Source: three-view drawing plus pictorial views. Frame: mm from the lowest corner of the part. A direction names the side the tool comes from. Give positions to 0.01 mm unless a question says otherwise; leave off trailing zeros. Loops run counter-clockwise (first coordinate to the right, second up) from the corner with the lowest first, then second, coordinate; pieces in that order, holes last. Notation, with made-up numbers: (74, 63) - (123, 63) arc R10 cw to (123, 68) - close; hole circle Ø7 at (-37, 78). An arc over 180 degrees is marked (long way). Answer as a JSON object with one key per item and string values. Group by question number.
(1) Section query B-B (y = 27.5). Return loops of the section in (x, z).
(2) Section query C-C (z = 7). Return loops of the section in (x, y).
(3) Section query D-D (x = 30). Return loops of the section in (y, z).
(4) Access query for the marked faces 1, 2, 3 and 4. Directions: +Z, -Z, +X, -X, +Y, -Y. A direction counts if a zero-diameter tool reaches every point of the face in a straight line with its end or side. Return the directions, or none.
(5) Pin query (flat end, axial travel): P1, Ø3, axis at y = 4, z = 5.5, coming from the +X side; P2, Ø1.5, axis at x = 26.5, z = 10.5, coming from the +Y side; P3, Ø6, axis at x = 30, y = 7.5, coming from the -Z side; P4, Ø3, axis at x = 16, z = 5, coming from the -Y side. Return the tip coordinate at first contact, or that it passes through.
(6) Mould query, pull axis X, two halves, no side actions, for the marked faces 5, 6, 7 and 8. Classes: +X half, -X half, draft (parallel to the pull), parting line (faces both ways), or undercut.
(7) Section query A-A (x = 12.5). Return loops of the section in (y, z), plus the area to 3 significant figures.
(8) Material intervals for L1, parallel to X at y = 16, z = 6.75; L2, parallel to Y at x = 12.5, z = 9.8; L3, parallel to Y at x = 30, z = 11.25, sorted ascending.
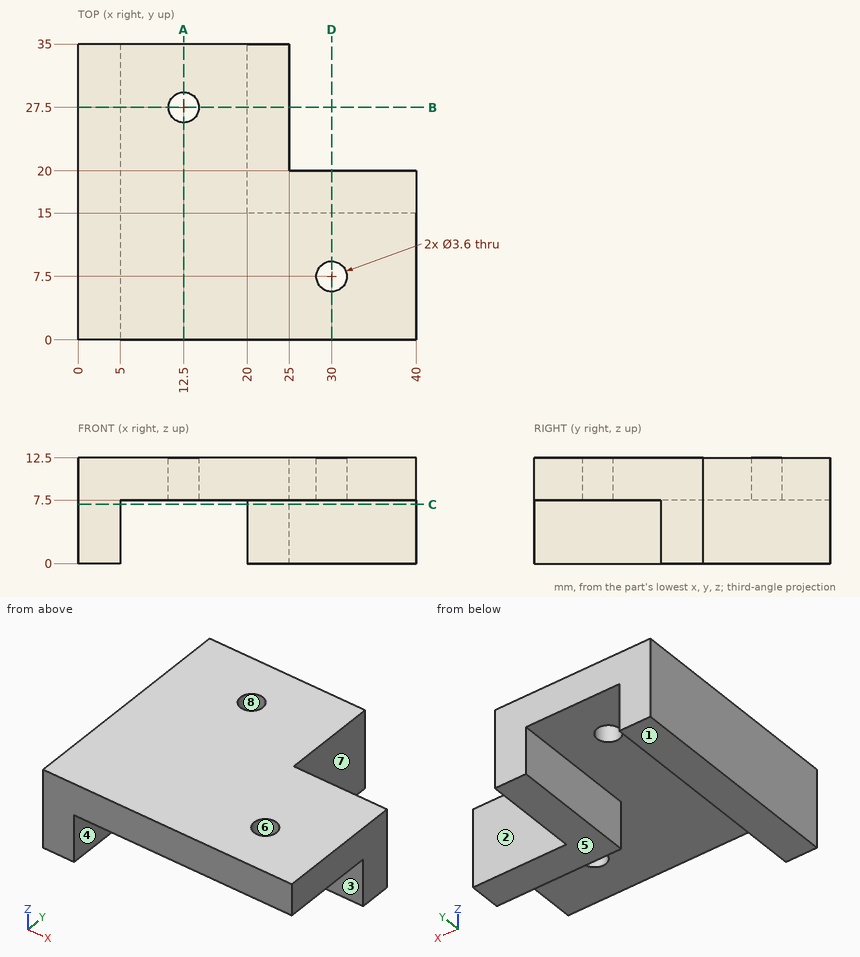
Recorded:
{
 "1": {"outline": "(0, 0) - (5, 0) - (5, 7.5) - (10.7, 7.5) - (10.7, 12.5) - (0, 12.5) - close; (14.3, 7.5) - (20, 7.5) - (20, 0) - (25, 0) - (25, 12.5) - (14.3, 12.5) - close"},
 "2": {"outline": "(0, 0) - (5, 0) - (5, 35) - (0, 35) - close; (20, 15) - (40, 15) - (40, 20) - (25, 20) - (25, 35) - (20, 35) - close"},
 "3": {"outline": "(0, 7.5) - (5.7, 7.5) - (5.7, 12.5) - (0, 12.5) - close; (9.3, 7.5) - (15, 7.5) - (15, 0) - (20, 0) - (20, 12.5) - (9.3, 12.5) - close"},
 "4": {"face 1": "-Z, +X, -X, +Y, -Y", "face 2": "+Z, -Z, +X, +Y", "face 3": "-Z, +X, -Y", "face 4": "-Z, +Y, -Y"},
 "5": {"P1": "stops at x = 5", "P2": "stops at y = 20", "P3": "stops at z = 7.5", "P4": "passes through"},
 "6": {"face 5": "draft", "face 6": "undercut", "face 7": "+X half", "face 8": "undercut"},
 "7": {"outline": "(0, 7.5) - (25.7, 7.5) - (25.7, 12.5) - (0, 12.5) - close; (29.3, 7.5) - (35, 7.5) - (35, 12.5) - (29.3, 12.5) - close", "area": "157 mm^2"},
 "8": {"L1": "x = 0 to 5, 20 to 40", "L2": "y = 0 to 25.7, 29.3 to 35", "L3": "y = 0 to 5.7, 9.3 to 20"}
}
